Solid Edge part; units mm, degrees
sketch "Sketch1" plane through (0, 0, 0) normal (0, 0, 1) x (1, 0, 0)
  line L0 (-25, 30) -> (-25, 0)
  line L1 (-25, 0) -> (25, 0)
  line L2 (25, 0) -> (25, 30)
  line L3 (10, 50) -> (25, 30)
  line L4 (-10, 50) -> (10, 50)
  line L5 (-25, 30) -> (-10, 50)
  dimension "D1" = 25
  dimension "D2" = 25
  dimension "D3" = 10
extrude "Protrusion1" add sketch "Sketch1" along normal mid plane 4
hole "Hole_1" at (-10, 40, 2) direction (0, 0, -1) diameter 4 end up to next
hole "Hole1" at (10, 40, 2) direction (0, 0, -1) diameter 4 end up to next
hole "Hole2" at (-20, 5, 2) direction (0, 0, -1) diameter 4 end up to next
hole "Hole3" at (20, 5, 2) direction (0, 0, -1) diameter 4 end up to next
chamfer "Chamfer_1" distance 1 angle 45 6 edges at (25, 15, -2) (17.5, 40, -2) (0, 50, -2) (-17.5, 40, -2) (-25, 15, -2) (0, 0, -2)
properties material "Polyethylene, low density"
Model file for the job. Use its own axes, mm. Round coordinates to 2 decimals unless told otherwise and drop trailing zeros. Loops run counter-clockwise (first coordinate to the right, second up) from the corner with the lowest first, then second, coordinate; pieces in that order, holes last.
1. Band-saw the part on C-C, the plane x = -19. List the corners of the cut face in (y, z).
Check values:
outline: (0, -1) - (1, -2) - (3.27, -2) - (3.27, 2) - (0, 2) - close; (6.73, -2) - (36.33, -2) - (38, -1) - (38, 2) - (6.73, 2) - close
2. Wall check: probe 1 along Y at (x, z) = (-10, 0.6); probe 2 along X at (y, z) = (5, -0.25); probe 3 along X at (y, z) = (40, 0.15). Give the ranges that are in metal, low to high.
Check values:
probe 1: y = 0 to 38, 42 to 50
probe 2: x = -25 to -22, -18 to 18, 22 to 25
probe 3: x = -17.5 to -12, -8 to 8, 12 to 17.5
3. Mould opens along Y. For faces 1 (the cylindrical face through (11.352, 41.474, 0.028)), 2 (the flat face through (-16.989, 39.836, -1.507)), 3 (the flat face through (0, 25, -2)), 4 (the flat face through (0, 0, 0)) say: +Y half, -Y half, draft (parallel to the pull), parting line (faces both ways), or undercut.
Check values:
face 1: undercut
face 2: +Y half
face 3: draft
face 4: -Y half
4. Band-saw the part on A-A, the plane y = 40. List the corners of the cut face in (x, z), and give its area (3 significant figures).
Check values:
outline: (-17.5, -1) - (-16.25, -2) - (-12, -2) - (-12, 2) - (-17.5, 2) - close; (-8, -2) - (8, -2) - (8, 2) - (-8, 2) - close; (12, -2) - (16.25, -2) - (17.5, -1) - (17.5, 2) - (12, 2) - close
area: 107 mm2
5. Band-saw the part on B-B, the plane z = 0.2. List the corners of the cut face in (x, y), and give its area (3 significant figures).
Check values:
outline: (-25, 0) - (25, 0) - (25, 30) - (10, 50) - (-10, 50) - (-25, 30) - close; hole circle Ø4 at (-20, 5); hole circle Ø4 at (-10, 40); hole circle Ø4 at (10, 40); hole circle Ø4 at (20, 5)
area: 2,150 mm2
6. Drop a flat-ended pin along its axis: P1, Ø5, axis at x = -10, y = 40, coming from the +Z side. Give the stop position or say it passes through.
Check values:
P1: stops at z = 2
7. Band-saw the part on D-D, the plane y = 5. List the corners of the cut face in (x, z), and give its area (3 significant figures).
Check values:
outline: (-25, -1) - (-24, -2) - (-22, -2) - (-22, 2) - (-25, 2) - close; (-18, -2) - (18, -2) - (18, 2) - (-18, 2) - close; (22, -2) - (24, -2) - (25, -1) - (25, 2) - (22, 2) - close
area: 167 mm2
